```python
from build123d import *

# Parameters (mm, degrees)
F1_DEPTH     = 3.81
F2_T1_DEPTH  = 139.7
F2_T3_DEPTH  = 63.5
F2_T6_ANGLE  = 90
F2_T8_ANGLE  = 90
F2_T10_ANGLE = 90
F2_T12_ANGLE = 90
F3_DEPTH     = 3.81
F4_T1_DEPTH  = 139.7
F4_T3_DEPTH  = 63.5
F4_T6_ANGLE  = 90
F4_T8_ANGLE  = 90
F4_T10_ANGLE = 90
F4_T12_ANGLE = 90


# Not quite as in the source:
# - a fillet or chamfer that OpenCascade refuses, or shapes differently, is made with other operations: its cross-section is extruded or revolved along the edge and cut away or added
# - the program builds the solid bodies; features that only make, move or delete a surface that nothing else refers to are left out


with BuildPart() as f1:
    # F0 (on Front) → F1 (new body)
    with BuildSketch(Plane.XZ):
        with BuildLine():
            Line((-31.75, -76.2), (31.75, -76.2))
            ThreePointArc((31.75, -76.2), (36.2401280605, -74.3401280605), (38.1, -69.85))
            Line((38.1, -69.85), (38.1, 69.85))
            ThreePointArc((38.1, 69.85), (36.2401280605, 74.3401280605), (31.75, 76.2))
            Line((31.75, 76.2), (-31.75, 76.2))
            ThreePointArc((-31.75, 76.2), (-36.2401280605, 74.3401280605), (-38.1, 69.85))
            Line((-38.1, 69.85), (-38.1, -69.85))
            ThreePointArc((-38.1, -69.85), (-36.2401280605, -74.3401280605), (-31.75, -76.2))
        make_face()
    extrude(amount=F1_DEPTH)

    # F2: fillet of radius 5.08 on 1 edges, made by hand

    # F2_s2 → F2_t1 (cut)
    with BuildSketch(Plane.XY.offset(-69.85)):
        with BuildLine():
            ThreePointArc((38.1, 0), (36.2921631237, -2.7460926284), (33.1813111503, -3.81))
            Line((33.1813111503, -3.81), (38.1, -3.81))
            Line((38.1, -3.81), (38.1, 0))
        make_face()
        with BuildLine():
            ThreePointArc((-38.1, 0), (-36.2921631237, -2.7460926284), (-33.1813111503, -3.81))
            Line((-33.1813111503, -3.81), (-38.1, -3.81))
            Line((-38.1, -3.81), (-38.1, 0))
        make_face()
    extrude(amount=F2_T1_DEPTH, mode=Mode.SUBTRACT)

    # F2_s4 → F2_t3 (cut)
    with BuildSketch(Plane.YZ.offset(-31.75)):
        with BuildLine():
            ThreePointArc((0, 76.2), (-2.7460926284, 74.3921631237), (-3.81, 71.2813111503))
            Line((-3.81, 71.2813111503), (-3.81, 76.2))
            Line((-3.81, 76.2), (0, 76.2))
        make_face()
        with BuildLine():
            ThreePointArc((0, -76.2), (-2.7460926284, -74.3921631237), (-3.81, -71.2813111503))
            Line((-3.81, -71.2813111503), (-3.81, -76.2))
            Line((-3.81, -76.2), (0, -76.2))
        make_face()
    extrude(amount=F2_T3_DEPTH, mode=Mode.SUBTRACT)

    # F2_s5 → F2_t6 (revolve, cut)
    with BuildSketch(Plane.YZ.offset(31.75)):
        with BuildLine():
            ThreePointArc((0, -76.2), (-2.7460926284, -74.3921631237), (-3.81, -71.2813111503))
            Line((-3.81, -71.2813111503), (-3.81, -76.2))
            Line((-3.81, -76.2), (0, -76.2))
        make_face()
    revolve(axis=Axis((31.75, -3.81, -69.85), (0, -1, 0)), revolution_arc=F2_T6_ANGLE, mode=Mode.SUBTRACT)

    # F2_s7 → F2_t8 (revolve, cut)
    with BuildSketch(Plane.XY.offset(69.85)):
        with BuildLine():
            ThreePointArc((38.1, 0), (36.2921631237, -2.7460926284), (33.1813111503, -3.81))
            Line((33.1813111503, -3.81), (38.1, -3.81))
            Line((38.1, -3.81), (38.1, 0))
        make_face()
    revolve(axis=Axis((31.75, -3.81, 69.85), (0, -1, 0)), revolution_arc=F2_T8_ANGLE, mode=Mode.SUBTRACT)

    # F2_s9 → F2_t10 (revolve, cut)
    with BuildSketch(Plane.YZ.offset(-31.75)):
        with BuildLine():
            ThreePointArc((0, 76.2), (-2.7460926284, 74.3921631237), (-3.81, 71.2813111503))
            Line((-3.81, 71.2813111503), (-3.81, 76.2))
            Line((-3.81, 76.2), (0, 76.2))
        make_face()
    revolve(axis=Axis((-31.75, -3.81, 69.85), (0, -1, 0)), revolution_arc=F2_T10_ANGLE, mode=Mode.SUBTRACT)

    # F2_s11 → F2_t12 (revolve, cut)
    with BuildSketch(Plane.XY.offset(-69.85)):
        with BuildLine():
            ThreePointArc((-38.1, 0), (-36.2921631237, -2.7460926284), (-33.1813111503, -3.81))
            Line((-33.1813111503, -3.81), (-38.1, -3.81))
            Line((-38.1, -3.81), (-38.1, 0))
        make_face()
    revolve(axis=Axis((-31.75, -3.81, -69.85), (0, -1, 0)), revolution_arc=F2_T12_ANGLE, mode=Mode.SUBTRACT)

    # F3 (add): a face of the model
    f3_faces = [f1.faces().sort_by_distance(p)[0] for p in [
        (0, 0, 0),
    ]]
    extrude(f3_faces, amount=F3_DEPTH)

    # F4: fillet of radius 5.08 on 1 edges, made by hand

    # F4_s2 → F4_t1 (cut)
    with BuildSketch(Plane.XY.offset(-69.85)):
        with BuildLine():
            ThreePointArc((33.1813111503, 3.81), (36.2921631237, 2.7460926284), (38.1, 0))
            Line((38.1, 0), (38.1, 3.81))
            Line((38.1, 3.81), (33.1813111503, 3.81))
        make_face()
        with BuildLine():
            ThreePointArc((-38.1, 0), (-36.2921631237, 2.7460926284), (-33.1813111503, 3.81))
            Line((-33.1813111503, 3.81), (-38.1, 3.81))
            Line((-38.1, 3.81), (-38.1, 0))
        make_face()
    extrude(amount=F4_T1_DEPTH, mode=Mode.SUBTRACT)

    # F4_s4 → F4_t3 (cut)
    with BuildSketch(Plane.YZ.offset(-31.75)):
        with BuildLine():
            ThreePointArc((3.81, 71.2813111503), (2.7460926284, 74.3921631237), (0, 76.2))
            Line((0, 76.2), (3.81, 76.2))
            Line((3.81, 76.2), (3.81, 71.2813111503))
        make_face()
        with BuildLine():
            ThreePointArc((3.81, -71.2813111503), (2.7460926284, -74.3921631237), (0, -76.2))
            Line((0, -76.2), (3.81, -76.2))
            Line((3.81, -76.2), (3.81, -71.2813111503))
        make_face()
    extrude(amount=F4_T3_DEPTH, mode=Mode.SUBTRACT)

    # F4_s5 → F4_t6 (revolve, cut)
    with BuildSketch(Plane.YZ.offset(31.75)):
        with BuildLine():
            ThreePointArc((3.81, -71.2813111503), (2.7460926284, -74.3921631237), (0, -76.2))
            Line((0, -76.2), (3.81, -76.2))
            Line((3.81, -76.2), (3.81, -71.2813111503))
        make_face()
    revolve(axis=Axis((31.75, 3.81, -69.85), (0, -1, 0)), revolution_arc=F4_T6_ANGLE, mode=Mode.SUBTRACT)

    # F4_s7 → F4_t8 (revolve, cut)
    with BuildSketch(Plane.XY.offset(69.85)):
        with BuildLine():
            ThreePointArc((33.1813111503, 3.81), (36.2921631237, 2.7460926284), (38.1, 0))
            Line((38.1, 0), (38.1, 3.81))
            Line((38.1, 3.81), (33.1813111503, 3.81))
        make_face()
    revolve(axis=Axis((31.75, 3.81, 69.85), (0, -1, 0)), revolution_arc=F4_T8_ANGLE, mode=Mode.SUBTRACT)

    # F4_s9 → F4_t10 (revolve, cut)
    with BuildSketch(Plane.YZ.offset(-31.75)):
        with BuildLine():
            ThreePointArc((0, 76.2), (2.7460926284, 74.3921631237), (3.81, 71.2813111503))
            Line((3.81, 71.2813111503), (3.81, 76.2))
            Line((3.81, 76.2), (0, 76.2))
        make_face()
    revolve(axis=Axis((-31.75, 3.81, 69.85), (0, -1, 0)), revolution_arc=F4_T10_ANGLE, mode=Mode.SUBTRACT)

    # F4_s11 → F4_t12 (revolve, cut)
    with BuildSketch(Plane.XY.offset(-69.85)):
        with BuildLine():
            ThreePointArc((-38.1, 0), (-36.2921631237, 2.7460926284), (-33.1813111503, 3.81))
            Line((-33.1813111503, 3.81), (-38.1, 3.81))
            Line((-38.1, 3.81), (-38.1, 0))
        make_face()
    revolve(axis=Axis((-31.75, 3.81, -69.85), (0, -1, 0)), revolution_arc=F4_T12_ANGLE, mode=Mode.SUBTRACT)


solid = f1.part
```
For this review, take the finished solid that the model builds, in its own axes (mm). Coordinates: 2 decimals unless noted, no trailing zeros. Loops run counter-clockwise (first coordinate to the right, second up) from the corner with the lowest first, then second, coordinate; pieces in that order, holes last. Notation, with made-up numbers: (82, 88) - (111, 88) arc R27 ccw to (111, 104) - close; hole circle Ø3 at (-14.5, -1.5). An arc over 180 degrees is marked (long way). Use one line per item in the form item = value. Start each with the question number.
1) To check wall thickness, follow probe 1 along X at (y, z) = (-1.75, 62); probe 2 along X at (y, z) = (-1.25, 28); probe 3 along Z at (x, y) = (24.5, 2.5). State the ranges of each line that lie inside material, in increasing order. Write a range as from..to.
2) Take a section at B-B (z = -58.5). State the section outline as (x, y) points, plus the area to 3 significant figures.
3) Take a section at A-A (x = -15). State the section outline as (y, z) points.
4) For pin 1 (3 mm diameter, centred on y = -2, z = -4.5, fed in from +X), flat-tipped, find the tip position at first contact; note if it passes through.
From the geometry:
q1.probe_1 = -37.27..37.27
q1.probe_2 = -37.59..37.59
q1.probe_3 = -74.69..74.69
q2.outline = (-38.1, 0) arc R5.08 ccw to (-33.18, -3.81) - (33.18, -3.81) arc R5.08 ccw to (38.1, 0) arc R5.08 ccw to (33.18, 3.81) - (-33.18, 3.81) arc R5.08 ccw to start
q2.area = 561 mm2
q3.outline = (-3.81, -71.28) arc R5.08 ccw to (0, -76.2) arc R5.08 ccw to (3.81, -71.28) - (3.81, 71.28) arc R5.08 ccw to (0, 76.2) arc R5.08 ccw to (-3.81, 71.28) - close
q4.pin_1 = 37.94
